Verification items for the finished model (mm, model axes). A direction names the side the tool comes from. Round coordinates to 2 decimals unless told otherwise and drop trailing zeros. One line per question, with ' | ' between items.
from build123d import *

# Parameters (mm, degrees)
CUT_EXTRUDE1_DEPTH = 51.813384221
SKETCH3_W          = 20.914953444
SKETCH3_H          = 10
CUT_EXTRUDE2_DEPTH = 51.813384221


with BuildPart() as part:
    # Sketch1 → Loft1 section 0
    with BuildSketch(Plane(origin=(0, 0, 0), x_dir=(1, 0, 0), z_dir=(0, 1, 0))):
        with BuildLine():
            Line((-25.17448832, 6.3), (-27.3, 3.111028865))
            Line((-27.3, 3.111028865), (-27.3, -3.111028865))
            Line((-27.3, -3.111028865), (-25.17448832, -6.3))
            Line((-25.17448832, -6.3), (-13.695486873, -6.3))
            Line((-13.695486873, -6.3), (13.695486873, -6.3))
            Line((13.695486873, -6.3), (24.588730163, -6.3))
            Line((24.588730163, -6.3), (27.3, -3.588730163))
            Line((27.3, -3.588730163), (27.3, 3.588730163))
            Line((27.3, 3.588730163), (24.588730163, 6.3))
            Line((24.588730163, 6.3), (13.695486873, 6.3))
            Line((13.695486873, 6.3), (-13.695486873, 6.3))
            Line((-13.695486873, 6.3), (-25.17448832, 6.3))
        make_face()
    # Sketch2 → Loft1 section 1
    with BuildSketch(Plane(origin=(0, -39, 0), x_dir=(1, 0, 0), z_dir=(0, 1, 0))):
        with BuildLine():
            Line((26.121320344, 10), (13.695486873, 10))
            Line((13.695486873, 10), (-13.695486873, 10))
            Line((-13.695486873, 10), (-27.154910603, 10))
            Line((-27.154910603, 10), (-31, 4.231093051))
            Line((-31, 4.231093051), (-31, -4.231093051))
            Line((-31, -4.231093051), (-27.154910603, -10))
            Line((-27.154910603, -10), (-13.695486873, -10))
            Line((-13.695486873, -10), (13.695486873, -10))
            Line((13.695486873, -10), (26.121320344, -10))
            Line((26.121320344, -10), (31, -5.121320344))
            Line((31, -5.121320344), (31, 5.121320344))
            Line((31, 5.121320344), (26.121320344, 10))
        make_face()
    loft()

    # Sketch1<4> → Cut-Extrude1 (cut, through all)
    with BuildSketch(Plane(origin=(0, 0, 0), x_dir=(1, 0, 0), z_dir=(0, 1, 0))):
        with BuildLine():
            ThreePointArc((21, 2.45), (18.55, 0), (21, -2.45))
            ThreePointArc((21, -2.45), (23.45, 0), (21, 2.45))
        make_face()
        with BuildLine():
            ThreePointArc((-21, -2.45), (-18.55, 0), (-21, 2.45))
            ThreePointArc((-21, 2.45), (-23.45, 0), (-21, -2.45))
        make_face()
    extrude(amount=-CUT_EXTRUDE1_DEPTH, mode=Mode.SUBTRACT)

    # Sketch3 → Cut-Extrude2 (cut, symmetric)
    with BuildSketch(Plane.XY):
        with Locations((-26.457476722, -20)):
            Rectangle(SKETCH3_W, SKETCH3_H)
    cut_extrude2 = extrude(amount=CUT_EXTRUDE2_DEPTH, both=True, mode=Mode.SUBTRACT)

    # Mirror1: Cut-Extrude2 across plane
    add(cut_extrude2.mirror(Plane(origin=(0, 0, 0), x_dir=(0, 0, 1), z_dir=(1, 0, 0))), mode=Mode.SUBTRACT)


solid = part.part
1. Mould release check, pull along Z, two halves, no side actions. Record for faces 4 (the face through (19.509, -7.395, -1.944)), 5 (the face through (-24, -15, 0)): pulls with the +Z half, pulls with the -Z half, needs draft (parallel to the pull), parting line crosses it, or undercut.
Results:
face 4: undercut | face 5: needs draft
2. Tool access check on faces 1 (the face through (-16, -20, 0)), 2 (the face through (0, -39, 0)), 3 (the face through (16, -20, 0)). Record the directions out of +Z, -Z, +X, -X, +Y, -Y that give a thin tool (end or side, any length) a straight path to the whole face; none if there is none.
Results:
face 1: +Z, -Z, -X | face 2: +Z, -Z, +X, -X, -Y | face 3: +Z, -Z, +X
3. Thickness scan on line 1 (Y direction, x = -16.5, z = -2.75); line 2 (X direction, y = -28, z = 2); line 3 (X direction, y = -23.5, z = 2.25). Record the ranges inside material, lowest first.
Results:
line 1: y = -39 to -25, -15 to 0 | line 2: x = -29.96 to -22.42, -19.58 to 19.58, 22.42 to 29.96 | line 3: x = -16 to 16
4. Section check A-A, the plane x = -21. Count the separate pieces of the cut face and the enclosed holes in it, then the cut area to 3 significant figures.
Results:
separate pieces: 4 | enclosed holes: 0 | area: 330 mm2
5. Go/stop test with flat-tipped pins: P1, Ø2, axis at x = -5, y = -28.5, coming from the -Z side; P2, Ø10, axis at x = -4.5, z = -3.5, coming from the +Y side; P3, Ø4, axis at x = 6.5, y = -21.5, coming from the -Z side; P4, Ø5, axis at y = -22, z = -1, coming from the +X side. Record where each tip stops, or that it passes through.
Results:
P1: stops at z = -9.1 | P2: stops at y = 0 | P3: stops at z = -8.53 | P4: stops at x = 16
